```python
from build123d import *

# Parameters (mm, degrees)
Y_KSEKLIK_EKSTR_ZYON1_DEPTH = 3
IZIM2_R                     = 1.5
KES_EKSTR_ZYON1_DEPTH       = 10
IZIM4_R                     = 1.5
KES_EKSTR_ZYON2_DEPTH       = 10


with BuildPart() as part:
    # Çizim1 → Yükseklik-Ekstrüzyon1 (new body)
    with BuildSketch(Plane(origin=(0, 0, 0), x_dir=(1, 0, 0), z_dir=(0, 1, 0))):
        with BuildLine():
            Line((3.903882032, 0), (112.096117968, 0))
            ThreePointArc((112.096117968, 0), (115.173179015, -1.05897281), (116.946830469, -3.787321875))
            Line((116.946830469, -3.787321875), (136.446830469, -81.787321875))
            ThreePointArc((136.446830469, -81.787321875), (135.537145158, -86.077061047), (131.596117968, -88))
            Line((131.596117968, -88), (96.903882032, -88))
            ThreePointArc((96.903882032, -88), (93.826820985, -86.94102719), (92.053169531, -84.212678125))
            Line((92.053169531, -84.212678125), (90.946830469, -79.787321875))
            ThreePointArc((90.946830469, -79.787321875), (89.173179015, -77.05897281), (86.096117968, -76))
            Line((86.096117968, -76), (29.903882032, -76))
            ThreePointArc((29.903882032, -76), (26.826820985, -77.05897281), (25.053169531, -79.787321875))
            Line((25.053169531, -79.787321875), (23.946830469, -84.212678125))
            ThreePointArc((23.946830469, -84.212678125), (22.173179015, -86.94102719), (19.096117968, -88))
            Line((19.096117968, -88), (-15.596117968, -88))
            ThreePointArc((-15.596117968, -88), (-19.537145158, -86.077061047), (-20.446830469, -81.787321875))
            Line((-20.446830469, -81.787321875), (-0.946830469, -3.787321875))
            ThreePointArc((-0.946830469, -3.787321875), (0.826820985, -1.05897281), (3.903882032, 0))
        make_face()
    extrude(amount=Y_KSEKLIK_EKSTR_ZYON1_DEPTH)

    # Çizim2 → Kes-Ekstrüzyon1 (cut)
    with BuildSketch(Plane(origin=(0, 3, 0), x_dir=(1, 0, 0), z_dir=(0, 1, 0))):
        with Locations(Location((5.6, -7.73, 0), (0, 0, 270))):
            Circle(IZIM2_R)
        with Locations(Location((110.4, -7.73, 0), (0, 0, 90))):
            Circle(IZIM2_R)
    extrude(amount=-KES_EKSTR_ZYON1_DEPTH, mode=Mode.SUBTRACT)

    # Çizim4 → Kes-Ekstrüzyon2 (cut)
    with BuildSketch(Plane(origin=(0, 3, 0), x_dir=(1, 0, 0), z_dir=(0, 1, 0))):
        with Locations(Location((-11.94, -80.5, 0), (0, 0, 270))):
            Circle(IZIM4_R)
        with Locations(Location((127.94, -80.5, 0), (0, 0, 90))):
            Circle(IZIM4_R)
    extrude(amount=-KES_EKSTR_ZYON2_DEPTH, mode=Mode.SUBTRACT)


solid = part.part
```
CAD build for the part. Positions are in the model's coordinates, mm. A direction names the side the tool comes from. Round coordinates to 2 decimals unless told otherwise and drop trailing zeros. Order: outer loops, then holes, each group sorted by start corner. A loop starts at its lowest first (then second) coordinate and runs counter-clockwise, first axis right, second up.
Item 1: Probe line 1 along X through (y, z) = (1.3, 7.73); line 2 along Z through (x, y) = (110.4, 1.1); line 3 along X through (y, z) = (0.7, 80.5) (3 decimals). List the from-to ranges inside material, lowest first.
Item 2: Pin check, flat tips, straight feed: pin 1 (1 mm diameter, centred on y = 0.5, z = 32.5, fed in from -X); pin 2 (1.5 mm diameter, centred on x = 81, y = 0.5, fed in from +Z). Stop position of each tip, or through.
Item 3: Saw through at C-C on z = 7.73. Write the cut outline in (x, y).
Item 4: Saw through at A-A on x = 5.6. Write the cut outline in (y, z).
Item 5: Saw through at D-D on x = 127.94. Write the cut outline in (y, z), then the cut area to 3 significant figures.
Item 6: Tool access for faces 4 (the face through (126.56, 1.48, 42.24)), 5 (the face through (89.21, 1.48, 77.09)): list every direction of +Z, -Z, +X, -X, +Y, -Y with a clear straight run to the whole face (end or side of a thin tool).
Item 7: Saw through at B-B on y = 1.3. Write the cut outline in (x, z), then the cut area to 3 significant figures.
Item 8: Mould opens along Z. For faces 1 (the face through (115.136, 1.479, 1.031)), 2 (the face through (58, 1, 76)), 3 (the face through (-11.49, 1.52, 81.93)) say: pulls with the +Z half, pulls with the -Z half, needs draft (parallel to the pull), parting line crosses it, or undercut.
Reported:
1. line 1: x = -1.93 to 4.1, 7.1 to 108.9, 111.9 to 117.93
1. line 2: z = 0 to 6.23, 9.23 to 88
1. line 3: x = -20.125 to -13.44, -10.44 to 24.875, 91.125 to 126.44, 129.44 to 136.125
2. pin 1: stops at x = -8.25
2. pin 2: stops at z = 76
3. outline: (-1.93, 0) - (4.1, 0) - (4.1, 3) - (-1.93, 3) - close; (7.1, 0) - (108.9, 0) - (108.9, 3) - (7.1, 3) - close; (111.9, 0) - (117.93, 0) - (117.93, 3) - (111.9, 3) - close
4. outline: (0, 0) - (3, 0) - (3, 6.23) - (0, 6.23) - close; (0, 9.23) - (3, 9.23) - (3, 88) - (0, 88) - close
5. outline: (0, 47.76) - (3, 47.76) - (3, 79) - (0, 79) - close; (0, 82) - (3, 82) - (3, 88) - (0, 88) - close
5. area: 112 mm2
6. face 4: -Z, +X, +Y, -Y
6. face 5: +Z, +Y, -Y
7. outline: (-20.45, 81.79) - (-0.95, 3.79) arc R5 ccw to (3.9, 0) - (112.1, 0) arc R5 ccw to (116.95, 3.79) - (136.45, 81.79) arc R5 ccw to (131.6, 88) - (96.9, 88) arc R5 ccw to (92.05, 84.21) - (90.95, 79.79) arc R5 cw to (86.1, 76) - (29.9, 76) arc R5 cw to (25.05, 79.79) - (23.95, 84.21) arc R5 ccw to (19.1, 88) - (-15.6, 88) arc R5 ccw to start; hole circle Ø3 at (-11.94, 80.5); hole circle Ø3 at (5.6, 7.73); hole circle Ø3 at (110.4, 7.73); hole circle Ø3 at (127.94, 80.5)
7. area: 11,300 mm2
8. face 1: pulls with the -Z half
8. face 2: pulls with the +Z half
8. face 3: undercut
